from build123d import *

# Parameters (mm, degrees)
EXTRUDE_1_DEPTH     = 10.4
CUT_EXTRUDE_1_DEPTH = 7.5
SKETCH_3_R          = 2.1
CUT_EXTRUDE_2_DEPTH = 1.9
SKETCH_4_R          = 1.2
CUT_EXTRUDE_3_DEPTH = 3.2
EXTRUDE_2_DEPTH     = 9.91
CUT_EXTRUDE_4_DEPTH = 10
CUT_EXTRUDE_5_DEPTH = 10


with BuildPart() as part:
    # 草图1 → 凸台-拉伸1 (new body)
    with BuildSketch(Plane(origin=(0, 0, 0), x_dir=(1, 0, 0), z_dir=(0, 1, 0))):
        with BuildLine():
            Line((-22.3, -22.35), (22.3, -22.35))
            ThreePointArc((22.3, -22.35), (23.714213562, -21.764213562), (24.3, -20.35))
            Line((24.3, -20.35), (24.3, 20.35))
            ThreePointArc((24.3, 20.35), (23.714213562, 21.764213562), (22.3, 22.35))
            Line((22.3, 22.35), (-22.3, 22.35))
            ThreePointArc((-22.3, 22.35), (-23.714213562, 21.764213562), (-24.3, 20.35))
            Line((-24.3, 20.35), (-24.3, -20.35))
            ThreePointArc((-24.3, -20.35), (-23.714213562, -21.764213562), (-22.3, -22.35))
        make_face()
    extrude(amount=EXTRUDE_1_DEPTH)

    # 草图2 → 切除-拉伸1 (cut)
    with BuildSketch(Plane(origin=(0, 10.4, 0), x_dir=(1, 0, 0), z_dir=(0, 1, 0))):
        with BuildLine():
            Line((-20.7, -20.75), (20.7, -20.75))
            ThreePointArc((20.7, -20.75), (22.114213562, -20.164213562), (22.7, -18.75))
            Line((22.7, -18.75), (22.7, 18.75))
            ThreePointArc((22.7, 18.75), (22.114213562, 20.164213562), (20.7, 20.75))
            Line((20.7, 20.75), (-20.7, 20.75))
            ThreePointArc((-20.7, 20.75), (-22.114213562, 20.164213562), (-22.7, 18.75))
            Line((-22.7, 18.75), (-22.7, -18.75))
            ThreePointArc((-22.7, -18.75), (-22.114213562, -20.164213562), (-20.7, -20.75))
        make_face()
    extrude(amount=-CUT_EXTRUDE_1_DEPTH, mode=Mode.SUBTRACT)

    # 草图3 → 切除-拉伸2 (cut)
    with BuildSketch(Plane.XZ):
        with Locations(Location((-19.5, -17.55, 0), (0, 0, 270))):
            Circle(SKETCH_3_R)
        with Locations(Location((-19.5, 17.55, 0), (0, 0, 270))):
            Circle(SKETCH_3_R)
        with Locations(Location((16.5, 17.55, 0), (0, 0, 270))):
            Circle(SKETCH_3_R)
    extrude(amount=-CUT_EXTRUDE_2_DEPTH, mode=Mode.SUBTRACT)

    # 草图4 → 切除-拉伸3 (cut)
    with BuildSketch(Plane.XZ):
        with Locations(Location((-19.5, 17.55, 0), (0, 0, 90))):
            Circle(SKETCH_4_R)
        with Locations(Location((-19.5, -17.55, 0), (0, 0, 270))):
            Circle(SKETCH_4_R)
        with Locations(Location((16.5, 17.55, 0), (0, 0, 270))):
            Circle(SKETCH_4_R)
    extrude(amount=-CUT_EXTRUDE_3_DEPTH, mode=Mode.SUBTRACT)

    # 草图5 → 凸台-拉伸2 (add)
    with BuildSketch(Plane(origin=(0, 2.9, 0), x_dir=(1, 0, 0), z_dir=(0, 1, 0))):
        with BuildLine():
            Line((-4, 20.75), (1, 20.75))
            Line((1, 20.75), (1, 18.75))
            ThreePointArc((1, 18.75), (0.853553391, 18.396446609), (0.5, 18.25))
            Line((0.5, 18.25), (-3.5, 18.25))
            ThreePointArc((-3.5, 18.25), (-3.853553391, 18.396446609), (-4, 18.75))
            Line((-4, 18.75), (-4, 20.75))
        make_face()
        with BuildLine():
            Line((-3.5, -18.25), (0.5, -18.25))
            ThreePointArc((0.5, -18.25), (0.853553391, -18.396446609), (1, -18.75))
            Line((1, -18.75), (1, -20.75))
            Line((1, -20.75), (-4, -20.75))
            Line((-4, -20.75), (-4, -18.75))
            ThreePointArc((-4, -18.75), (-3.853553391, -18.396446609), (-3.5, -18.25))
        make_face()
    extrude(amount=EXTRUDE_2_DEPTH)

    # 草图6 → 切除-拉伸4 (cut)
    with BuildSketch(Plane.XZ):
        with BuildLine():
            Line((-12.821321535, 13), (-12.821321535, -13))
            ThreePointArc((-12.821321535, -13), (-13.821321535, -14), (-14.821321535, -13))
            Line((-14.821321535, -13), (-14.821321535, 13))
            ThreePointArc((-14.821321535, 13), (-13.821321535, 14), (-12.821321535, 13))
        make_face()
        with BuildLine():
            Line((-10, -12), (10, -12))
            ThreePointArc((10, -12), (11, -13), (10, -14))
            Line((10, -14), (-10, -14))
            ThreePointArc((-10, -14), (-11, -13), (-10, -12))
        make_face()
        with BuildLine():
            Line((12.821321535, 13), (12.821321535, -13))
            ThreePointArc((12.821321535, -13), (13.821321535, -14), (14.821321535, -13))
            Line((14.821321535, -13), (14.821321535, 13))
            ThreePointArc((14.821321535, 13), (13.821321535, 14), (12.821321535, 13))
        make_face()
        with BuildLine():
            Line((-10, 12), (10, 12))
            ThreePointArc((10, 12), (11, 13), (10, 14))
            Line((10, 14), (-10, 14))
            ThreePointArc((-10, 14), (-11, 13), (-10, 12))
        make_face()
    extrude(amount=-CUT_EXTRUDE_4_DEPTH, mode=Mode.SUBTRACT)

    # 草图7 → 切除-拉伸5 (cut)
    with BuildSketch(Plane.ZY.offset(24.3)):
        with BuildLine():
            Line((3.55, 10.4), (13.75, 10.4))
            Line((13.75, 10.4), (13.75, 9.9))
            ThreePointArc((13.75, 9.9), (13.603553391, 9.546446609), (13.25, 9.4))
            Line((13.25, 9.4), (4.05, 9.4))
            ThreePointArc((4.05, 9.4), (3.696446609, 9.546446609), (3.55, 9.9))
            Line((3.55, 9.9), (3.55, 10.4))
        make_face()
    extrude(amount=-CUT_EXTRUDE_5_DEPTH, mode=Mode.SUBTRACT)


solid = part.part
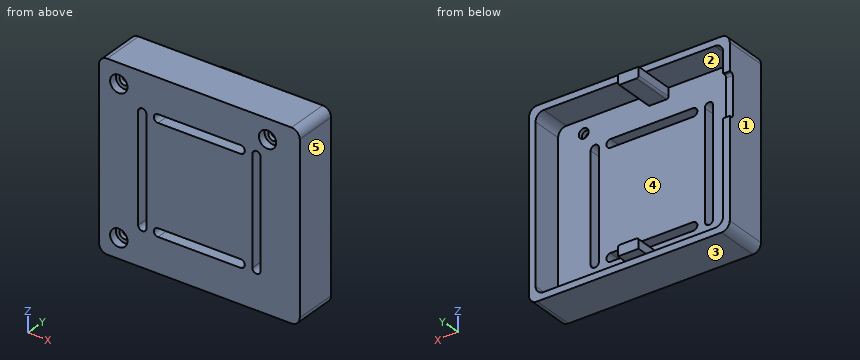
Build history of the part. All positions in model axes, mm. Face numbers are marked on the shaded views. A direction names the side the tool comes from. Coordinates: 2 decimals unless noted, no trailing zeros. Write each loop counter-clockwise with the first axis right and the second up, starting at its lowest first coordinate (ties: lowest second). Pieces come first, ordered by that corner, then holes.
(1) Pin check, flat tips, straight feed: pin 1 Ø22.5 at (x, z) = (7.5, -5.5) entering from +Y; pin 2 Ø3.5 at (x, z) = (-19.5, -17.55) entering from -Y. Stop position of each tip, or through.
(2) Drill centre lines: line 1 (X direction, y = 2.3, z = 17.55); line 2 (X direction, y = 1.3, z = 17.55); line 3 (Z direction, x = -10, y = 1). Where is each one in solid material? Low to high.
(3) Cut at C-C on y = 3.5. List the corners of the cut face in (x, z).
(4) 3-axis set-ups, long thin cutter, end or side, ignore diameter. For the marked faces 4 and 5: which of +Z, -Z, +X, -X, +Y, -Y reach the whole face in a straight line?
(5) Cut at D-D on x = 16.5. List the corners of the cut face in (y, z), and give its area (3 significant figures).
(6) Cut at A-A on z = 6. List the corners of the cut face in (x, y), and give its area (3 significant figures).
(7) Cut at B-B on x = -2. List the corners of the cut face in (y, z), and give its area (3 significant figures).
(8) Mould opens along Z. For the marked faces 1, 2 and 3 say: pulls with the +Z half, pulls with the -Z half, needs draft (parallel to the pull), parting line crosses it, or undercut.
Working result:
1. pin 1: stops at y = 2.9
1. pin 2: stops at y = 1.9
2. line 1: x = -24.3 to -20.7, -18.3 to 15.3, 17.7 to 24.3
2. line 2: x = -24.3 to -21.6, -17.4 to 14.4, 18.6 to 24.3
2. line 3: z = -22.35 to -14, -12 to 12, 14 to 22.35
3. outline: (-24.3, -20.35) arc R2 ccw to (-22.3, -22.35) - (22.3, -22.35) arc R2 ccw to (24.3, -20.35) - (24.3, 20.35) arc R2 ccw to (22.3, 22.35) - (-22.3, 22.35) arc R2 ccw to (-24.3, 20.35) - close; hole (-22.7, -18.75) arc R2 ccw to (-20.7, -20.75) - (-4, -20.75) - (-4, -18.75) arc R0.5 cw to (-3.5, -18.25) - (0.5, -18.25) arc R0.5 cw to (1, -18.75) - (1, -20.75) - (20.7, -20.75) arc R2 ccw to (22.7, -18.75) - (22.7, 18.75) arc R2 ccw to (20.7, 20.75) - (1, 20.75) - (1, 18.75) arc R0.5 cw to (0.5, 18.25) - (-3.5, 18.25) arc R0.5 cw to (-4, 18.75) - (-4, 20.75) - (-20.7, 20.75) arc R2 ccw to (-22.7, 18.75) - close
4. face 4: +Y
4. face 5: +Z, -Z, +X, +Y, -Y
5. outline: (0, -22.35) - (10.4, -22.35) - (10.4, -20.75) - (2.9, -20.75) - (2.9, 16.35) - (1.9, 16.35) - (1.9, 15.45) - (0, 15.45) - close; (0, 19.65) - (1.9, 19.65) - (1.9, 18.75) - (2.9, 18.75) - (2.9, 20.75) - (10.4, 20.75) - (10.4, 22.35) - (0, 22.35) - close
5. area: 143 mm2
6. outline: (-24.3, 0) - (-14.82, 0) - (-14.82, 2.9) - (-22.7, 2.9) - (-22.7, 9.4) - (-24.3, 9.4) - close; (-12.82, 0) - (12.82, 0) - (12.82, 2.9) - (-12.82, 2.9) - close; (14.82, 0) - (24.3, 0) - (24.3, 10.4) - (22.7, 10.4) - (22.7, 2.9) - (14.82, 2.9) - close
6. area: 152 mm2
7. outline: (0, -22.35) - (10.4, -22.35) - (10.4, -20.75) - (12.81, -20.75) - (12.81, -18.25) - (2.9, -18.25) - (2.9, -14) - (0, -14) - close; (0, -12) - (2.9, -12) - (2.9, 12) - (0, 12) - close; (0, 14) - (2.9, 14) - (2.9, 18.25) - (12.81, 18.25) - (12.81, 20.75) - (10.4, 20.75) - (10.4, 22.35) - (0, 22.35) - close
7. area: 192 mm2
8. face 1: needs draft
8. face 2: undercut
8. face 3: pulls with the -Z half
